Design review of the part built by this model. Coordinates are the model's own, in mm. A direction names the side the tool comes from. Round coordinates to 2 decimals unless told otherwise and drop trailing zeros. Loops run counter-clockwise (first coordinate to the right, second up) from the corner with the lowest first, then second, coordinate; pieces in that order, holes last. Notation, with made-up numbers: (48.25, -22.75) -> (106.25, -22.75) arc R30 ccw to (106.25, 1.25) -> close; hole circle Ø10 at (84, 75). An arc over 180 degrees is marked (long way). Use a Markdown table: item, result. Add a question column.
from build123d import *

# Parameters (mm, degrees)
SKETCH1_W           = 25.4
SKETCH1_H           = 12.7
BOSS_EXTRUDE1_DEPTH = 50.8
SHELL1_T            = -1.27


with BuildPart() as part:
    # Sketch1 → Boss-Extrude1 (new body)
    with BuildSketch(Plane.XY):
        Rectangle(SKETCH1_W, SKETCH1_H)
    extrude(amount=BOSS_EXTRUDE1_DEPTH)

    # Shell1
    shell1_openings = [part.faces().sort_by_distance(p)[0] for p in [
        (0, 0, 50.8),
        (-12.7, 0, 25.4),
        (0, 6.35, 25.4),
        (12.7, 0, 25.4),
    ]]
    offset(amount=SHELL1_T, openings=shell1_openings, kind=Kind.INTERSECTION)


solid = part.part
1. Consider section C-C on y = -1.5. State the section outline as (x, z) points, plus the area to 3 significant figures.
2. To check wall thickness, follow probe 1 along Y at (x, z) = (-6.5, 48.5); probe 2 along Z at (x, y) = (-4.5, -2). State the ranges of each line that lie inside material, in increasing order. Write a range as from..to.
3. Consider section A-A on x = -11. State the section outline as (y, z) points.
4. Insertion check: P1, Ø1.5, axis at x = 8, z = 18, coming from the +Y side; P2, Ø3, axis at x = -7.5, y = 2, coming from the +Z side; P3, Ø2, axis at x = -8, y = -2.5, coming from the -Z side. Each pin has a flat end and moves straight along its axis. Give the tip position at first contact, or say it passes through.
5. For faces 1 (the face through (0, -6, 50.8)), 2 (the face through (0, 1, 1.27)), list the 3-axis set-ups (+Z, -Z, +X, -X, +Y, -Y) from which the entire face can be reached by the end or side of a thin tool; tool diameter is ignored.
6. Consider section B-B on z = 39. State the section outline as (x, y) points.
Verdict:
| question | item | result |
|---|---|---|
| 1 | outline | (-12.7, 0) -> (12.7, 0) -> (12.7, 1.27) -> (-12.7, 1.27) -> close |
| 1 | area | 32.3 mm² |
| 2 | probe 1 | y = -6.35..-5.08 |
| 2 | probe 2 | z = 0..1.27 |
| 3 | outline | (-6.35, 0) -> (6.35, 0) -> (6.35, 1.27) -> (-5.08, 1.27) -> (-5.08, 50.8) -> (-6.35, 50.8) -> close |
| 4 | P1 | stops at y = -5.08 |
| 4 | P2 | stops at z = 1.27 |
| 4 | P3 | stops at z = 0 |
| 5 | face 1 | +Z, +X, -X, +Y, -Y |
| 5 | face 2 | +Z, +X, -X, +Y |
| 6 | outline | (-12.7, -6.35) -> (12.7, -6.35) -> (12.7, -5.08) -> (-12.7, -5.08) -> close |
